```python
from build123d import *

# Parameters (mm, degrees)
SKETCH_1_R      = 3
EXTRUDE_1_DEPTH = 3


with BuildPart() as part:
    # 草图1 → 凸台-拉伸1 (new body)
    with BuildSketch(Plane.XY):
        with BuildLine():
            Line((8.44582472, 166.89164944), (15, 180))
            ThreePointArc((15, 180), (30, 189.270509831), (45, 180))
            Line((45, 180), (51.55417528, 166.89164944))
            ThreePointArc((51.55417528, 166.89164944), (57.859919157, 149.494795444), (60, 131.1145618))
            Line((60, 131.1145618), (60, 0))
            Line((60, 0), (0, 0))
            Line((0, 0), (0, 10))
            ThreePointArc((0, 10), (-10.668063464, 65.5572809), (0, 121.1145618))
            Line((0, 121.1145618), (0, 131.1145618))
            ThreePointArc((0, 131.1145618), (2.140080843, 149.494795444), (8.44582472, 166.89164944))
        make_face()
        with Locations((50, 10)):
            Circle(SKETCH_1_R, mode=Mode.SUBTRACT)
        with Locations((30, 180)):
            Circle(SKETCH_1_R, mode=Mode.SUBTRACT)
        with Locations((10, 10)):
            Circle(SKETCH_1_R, mode=Mode.SUBTRACT)
    extrude(amount=EXTRUDE_1_DEPTH)


solid = part.part
```
Geometry: final body of the model. Coordinates: model frame, mm. Round coordinates to 2 decimals unless told otherwise and drop trailing zeros. Write each loop counter-clockwise with the first axis right and the second up, starting at its lowest first coordinate (ties: lowest second). Pieces come first, ordered by that corner, then holes.
Item 1: Section query A-A (x = 30). Return loops of the section in (y, z).
Item 2: Section query D-D (y = 126). Return loops of the section in (x, z).
Item 3: Pin query (flat end, axial travel): P1, Ø5, axis at x = 50, y = 10, coming from the +Z side; P2, Ø1.5, axis at y = 5, z = 2, coming from the -X side; P3, Ø12, axis at x = 20, y = 163, coming from the -Z side; P4, Ø1.5, axis at x = 46.5, z = 1, coming from the +Y side. Return the tip coordinate at first contact, or that it passes through.
Item 4: Section query C-C (x = 10.5). Return loops of the section in (y, z).
Item 5: Mould query, pull axis Y, two halves, no side actions, for faces 1 (the face through (29.74, 189.27, 1.48)), 2 (the face through (12.77, 8.85, 1.48)), 3 (the face through (25, 96, 0)), 4 (the face through (30, 183, 1)). Classes: +Y half, -Y half, draft (parallel to the pull), parting line (faces both ways), or undercut.
Item 6: Section query B-B (z = 1.15). Return loops of the section in (x, y).
Item 7: Material intervals for L1, parallel to X at y = 180, z = 1.2; L2, parallel to Y at x = 9.5, z = 1.55; L3, parallel to Y at x = 12.5, z = 1.3, sorted ascending.
Completed:
1. outline: (0, 0) - (177, 0) - (177, 3) - (0, 3) - close; (183, 0) - (189.27, 0) - (189.27, 3) - (183, 3) - close
2. outline: (0, 0) - (60, 0) - (60, 3) - (0, 3) - close
3. P1: passes through
3. P2: stops at x = 0
3. P3: stops at z = 0
3. P4: stops at y = 178.5
4. outline: (0, 0) - (7.04, 0) - (7.04, 3) - (0, 3) - close; (12.96, 0) - (171, 0) - (171, 3) - (12.96, 3) - close
5. face 1: +Y half
5. face 2: undercut
5. face 3: draft
5. face 4: undercut
6. outline: (0, 0) - (60, 0) - (60, 131.11) arc R80 ccw to (51.55, 166.89) - (45, 180) arc R16.77 ccw to (15, 180) - (8.45, 166.89) arc R80 ccw to (0, 131.11) - (0, 121.11) arc R150 ccw to (0, 10) - close; hole circle Ø6 at (10, 10); hole circle Ø6 at (30, 180); hole circle Ø6 at (50, 10)
7. L1: x = 15 to 27, 33 to 45
7. L2: y = 0 to 7.04, 12.96 to 169
7. L3: y = 0 to 8.34, 11.66 to 175
